The model under review builds one solid part; all positions refer to its coordinate system, in mm. Face numbers are marked on the shaded views. A direction names the side the tool comes from. Coordinates: 2 decimals unless noted, no trailing zeros. Order: outer loops, then holes, each group sorted by start corner. A loop starts at its lowest first (then second) coordinate and runs counter-clockwise, first axis right, second up. Notation, with made-up numbers: (-11, 56.25) -> (35, 56.25) arc R33 cw to (35, 95.25) -> close; hole circle Ø5 at (29, 62.25). An arc over 180 degrees is marked (long way). Put each result on its own line as item: value.
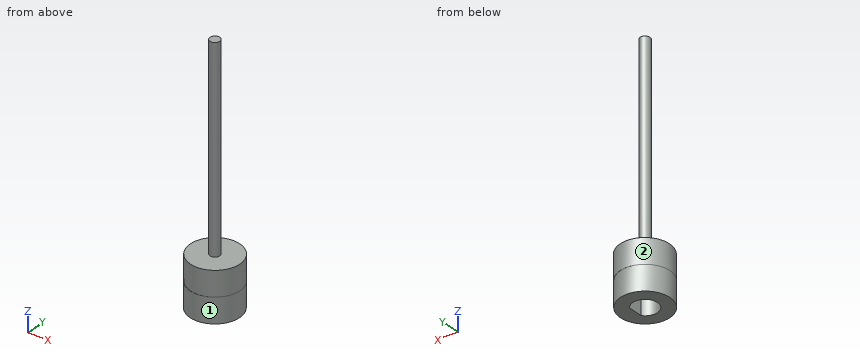
from build123d import *

# Parameters (mm, degrees)
SKETCH8_R           = 5
BOSS_EXTRUDE3_DEPTH = 5
SKETCH9_R           = 4.996260813
BOSS_EXTRUDE4_DEPTH = 5
SKETCH10_R          = 1
BOSS_EXTRUDE5_DEPTH = 40


with BuildPart() as part:
    # Sketch8 → Boss-Extrude3 (new body)
    with BuildSketch(Plane.XY):
        with Locations((-48.452108999, 26.292732134)):
            Circle(SKETCH8_R)
        with BuildLine():
            Line((-46.454907961, 26.292732134), (-46.454907961, 27.796456848))
            ThreePointArc((-46.454907961, 27.796456848), (-50.952108999, 26.292732134), (-46.454907961, 24.789007421))
            Line((-46.454907961, 24.789007421), (-46.454907961, 26.292732134))
        make_face(mode=Mode.SUBTRACT)
    extrude(amount=BOSS_EXTRUDE3_DEPTH)

    # Sketch9 → Boss-Extrude4 (add)
    with BuildSketch(Plane.XY.offset(5)):
        with Locations((-48.416448045, 26.317478542)):
            Circle(SKETCH9_R)
    extrude(amount=BOSS_EXTRUDE4_DEPTH)

    # Sketch10 → Boss-Extrude5 (add)
    with BuildSketch(Plane.XY.offset(10)):
        with Locations((-48.460247299, 26.321784668)):
            Circle(SKETCH10_R)
    extrude(amount=BOSS_EXTRUDE5_DEPTH)


solid = part.part
Item 1: For pin 1 Ø1.5 at (x, z) = (-45.5, 14.5) entering from -Y; pin 2 Ø3 at (x, y) = (-49, 26) entering from -Z; pin 3 Ø5 at (x, z) = (-46.5, 27.5) entering from -Y; pin 4 Ø5 at (x, y) = (-52, 26) entering from +Z, all flat-tipped, find the tip position at first contact; note any pin that passes through.
Answers below:
pin 1: through
pin 2: z = 5
pin 3: y = 25.32
pin 4: z = 10
Item 2: Consider section C-C on z = 8. Write out the cut boundary in (x, y), and give its area (3 significant figures).
Answers below:
outline: circle Ø9.99 at (-48.42, 26.32)
area: 78.4 mm^2
Item 3: For line 1 (Z direction, x = -51, y = 24); line 2 (Z direction, x = -48.5, y = 24.5); line 3 (Y direction, x = -50, z = 2), list the stretches that pass through material, from the lowest coordinate up. Write a range as from..to.
Answers below:
line 1: 0..10
line 2: 5..10
line 3: 21.54..24.33, 28.26..31.05
Item 4: For the marked faces 1 and 2, list the 3-axis set-ups (+Z, -Z, +X, -X, +Y, -Y) from which the entire face can be reached by the end or side of a thin tool; tool diameter is ignored.
Answers below:
face 1: -Z
face 2: +Z
